For this review, take the finished solid that the model builds, in its own axes (mm). Face numbers are marked on the shaded views. A direction names the side the tool comes from. Give positions to 0.01 mm unless a question says otherwise; leave off trailing zeros. Write each loop counter-clockwise with the first axis right and the second up, starting at its lowest first coordinate (ties: lowest second). Pieces come first, ordered by that corner, then holes. Notation, with made-up numbers: M 74.25,-22.75 L 86.25,-22.75 A32 cw 86.25,16.25 Z; hole C 4.5,77 d4. An arc over 180 degrees is marked long. Use one line per item in the form item = value. Start each with the question number.
Q1. Consider section D-D on x = -19.5. Write out the cut boundary in (y, z).
Q2. Consider section B-B on y = 16. Write out the cut boundary in (x, z), and give its area (3 significant figures).
Q3. For probe 1 along Z at (x, y) = (-7, 1.5); probe 2 along Z at (x, y) = (18, 6); probe 3 along Y at (x, z) = (28.75, -25), list the stretches that pass through material, from the lowest coordinate up. Write a range as [from, to].
Q4. Clearance check with flat-ended pins moving along their axes: pin 1 Ø1.5 at (y, z) = (38.5, -2) entering from +X; pin 2 Ø4 at (x, z) = (-7, 12.5) entering from -Y; pin 3 Ø6 at (y, z) = (42.5, -2.5) entering from -X; pin 4 Ø2 at (x, z) = (18, 11.5) entering from +Y. State where each tip first meets the part, or that it passes through.
Q5. Consider section A-A on z = -12.5. Write out the cut boundary in (x, y).
Q6. Tool access review of the marked faces 1, 2 and 3: name each direction out of +Z, -Z, +X, -X, +Y, -Y from which nothing blocks a thin tool from reaching the whole face with its end or side.
Q7. Consider section C-C on z = -25. Write out the cut boundary in (x, y), and give its area (3 significant figures).
Q8. Mouldability with a two-part tool opening along Z and no side actions: class the marked faces 4, 5, 6 and 7 as released by +Z, released by -Z, zero draft, split by the parting line, or undercut.
Autodesk Inventor part; units mm, degrees
ref_plane "YZ Plane" through (0, 0, 0) normal (1, 0, 0) x (0, 1, 0)
ref_plane "XZ Plane" through (0, 0, 0) normal (0, 1, 0) x (-1, 0, 0)
ref_plane "XY Plane" through (0, 0, 0) normal (0, 0, 1) x (1, 0, 0)
sketch "Skizze1" plane through (0, 0, 0) normal (0, 1, 0) x (-1, 0, 0)
  line L0 (-30, 30) -> (30, 30)
  line L1 (30, 30) -> (30, -30)
  line L2 (30, -30) -> (-30, -30)
  line L3 (-30, -30) -> (-30, 30)
  line L4 (-30, 30) -> (30, -30) construction
  line L5 (30, 30) -> (-30, -30) construction
  point P0 (0, 0)
  dimension "d0" = 60
  dimension "d1" = 60
extrude "Extrusion1" add sketch "Skizze1" along normal blind 8
sketch "Skizze2" plane through (0, 8, 0) normal (0, 1, 0) x (1, 0, 0)
  line L0 (-30, -30) -> (30, -30)
  line L1 (30, 30) -> (-30, 30)
  line L2 (30, -30) -> (22, -30)
  line L3 (22, -30) -> (22, 30)
  line L4 (22, 30) -> (30, 30)
  line L5 (30, 30) -> (30, -30)
  point P0 (0, 0)
  dimension "d4" = 8
extrude "Extrusion2" add sketch "Skizze2" along normal blind 40
sketch "Skizze3" plane through (0, 8, 0) normal (0, 1, 0) x (1, 0, 0)
  line L0 (42, 0) -> (-42, 0)
  line L1 (22, 30) -> (22, -30)
  point P0 (0, 0)
  point P1 (18, -12.5)
  point P2 (18, 12.5)
  point P3 (-7, 12.5)
  point P4 (-7, -12.5)
  dimension "d7" = 25
  dimension "d8" = 25
  dimension "d9" = 4
hole "Bohrung1" at (18, 8, 12.5) at (18, 8, -12.5) at (-7, 8, -12.5) at (-7, 8, 12.5) direction (0, -1, 0) diameter 3.4 end through all counterbore diameter 6.5 counterbore depth 3.4
sketch "Skizze4" plane through (30, 0, 30) normal (1, 0, 0) x (0, 0, -1)
  line L0 (30, -9.6) -> (30, 57.6)
  circle A0 centre (5, 5) radius 2
  circle A1 centre (55, 5) radius 2
  line L1 (0, 48) -> (60, 48)
  line L2 (0, 0) -> (60, 0)
  circle A2 centre (55, 30) radius 2
  circle A3 centre (5, 30) radius 2
  point P0 (30, 0)
  dimension "d17" = 4
  dimension "d18" = 50
  dimension "d22" = 5
  dimension "d25" = 25
extrude "Extrusion3" cut sketch "Skizze4" against normal blind 7
sketch "Skizze5" plane through (0, 0, 0) normal (0, 0, 1) x (1, 0, 0)
  line L0 (30, 48) -> (22, 48)
  line L1 (-30, 0) -> (-30, 8)
  line L2 (22, 48) -> (-30, 8)
  line L3 (-30, 8) -> (22, 8)
  line L4 (22, 8) -> (22, 48)
  point P0 (0, 0)
extrude "Extrusion4" add sketch "Skizze5" against normal blind 6 from surface at 30
mirror "Spiegeln1" about plane through (0, 0, 0) normal (0, 0, 1) of "Extrusion4"
sketch "Skizze6" plane through (0, 48, 0) normal (0, 1, 0) x (1, 0, 0)
  line L0 (33, -6.5) -> (27, -6.5)
  line L1 (27, -6.5) -> (27, 6.5)
  line L2 (27, 6.5) -> (33, 6.5)
  line L3 (33, 6.5) -> (33, -6.5)
  line L4 (30, -30) -> (30, 30)
  line L5 (33, -6.5) -> (27, 6.5) construction
  line L6 (27, -6.5) -> (33, 6.5) construction
  point P0 (0, 0)
  point P1 (30, 0)
  point P2 (30, -6.5)
  point P3 (30, 6.5)
  dimension "d26" = 3
  dimension "d27" = 13
extrude "Extrusion5" cut sketch "Skizze6" against normal through all contours L0 L1 L2 L4
sketch "Skizze7" plane through (0, 8, 0) normal (0, 1, 0) x (1, 0, 0)
  line L0 (-25, 16.1375) -> (-16, 16.1375) construction
  line L1 (-25, 13.3875) -> (-16, 13.3875)
  line L2 (-16, 18.8875) -> (-25, 18.8875)
  arc A0 (-25, 18.8875) -> (-25, 13.3875) centre (-25, 16.1375) ccw
  arc A1 (-16, 13.3875) -> (-16, 18.8875) centre (-16, 16.1375) ccw
  line L3 (-30, 24) -> (-30, -24)
  point P0 (0, 0)
  point P1 (-20.5, 16.1375)
  dimension "d30" = 5.5
  dimension "d31" = 9
  dimension "d32" = 9.5
extrude "Extrusion6" cut sketch "Skizze7" against normal through all
mirror "Spiegeln2" about plane through (0, 0, 0) normal (0, 0, 1) of "Extrusion6"
fillet "Rundung1" radius 4 4 edges at (26, 48, 30) (26, 48, -30) (-30, 4, 30) (-30, 4, -30)
properties part number "26_Laser_carriage_V2" material "PET-Kunststoff"
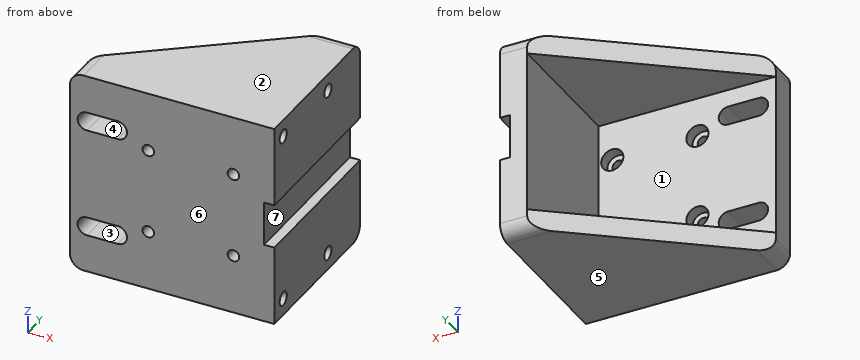
Working result:
q1.outline = M 0,-30 L 16.08,-30 L 16.08,-24 L 8,-24 L 8,-18.89 L 0,-18.89 Z; M 0,-13.39 L 8,-13.39 L 8,13.39 L 0,13.39 Z; M 0,18.89 L 8,18.89 L 8,24 L 16.08,24 L 16.08,30 L 0,30 Z
q2.outline = M -19.6,-30 L 30,-30 L 30,-6.5 L 27,-6.5 L 27,6.5 L 30,6.5 L 30,30 L -19.6,30 L -19.6,24 L 22,24 L 22,-24 L -19.6,-24 Z
q2.area = 940 mm²
q3.probe_1 = [-30, -14.2], [-10.8, 10.8], [14.2, 30]
q3.probe_2 = [-30, -15.75], [-9.25, 9.25], [15.75, 30]
q3.probe_3 = [0, 3], [7, 28], [32, 48]
q4.pin_1 = 27
q4.pin_2 = 0
q4.pin_3 = 22
q4.pin_4 = 4.6
q5.outline = M -30,0 L -8.7,0 L -8.7,4.6 L -10.25,4.6 L -10.25,8 L -30,8 Z; M -5.3,0 L 16.3,0 L 16.3,4.6 L 14.75,4.6 L 14.75,8 L -3.75,8 L -3.75,4.6 L -5.3,4.6 Z; M 19.7,0 L 30,0 L 30,48 L 22,48 L 22,8 L 21.25,8 L 21.25,4.6 L 19.7,4.6 Z
q6.face_1 = -X, +Y
q6.face_2 = +Z, +X, -X, +Y, -Y
q6.face_3 = +Y, -Y
q7.outline = M -30,0 L 30,0 L 30,3 L 23,3 L 23,7 L 30,7 L 30,28 L 23,28 L 23,32 L 30,32 L 30,48 L 22,48 L -30,8 Z
q7.area = 1,780 mm²
q8.face_4 = undercut
q8.face_5 = released by -Z
q8.face_6 = zero draft
q8.face_7 = undercut
